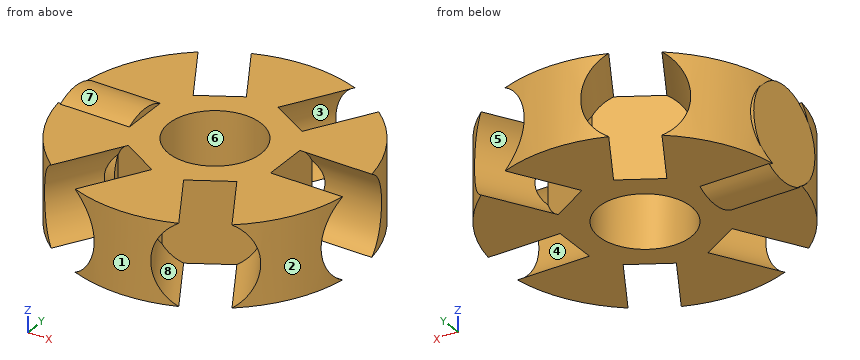
```python
from build123d import *

# Parameters (mm, degrees)
SKETCH1_R           = 12.5
SKETCH1_R_2         = 4
BOSS_EXTRUDE1_DEPTH = 3.5
SKETCH2_R           = 4
CUT_EXTRUDE3_DEPTH  = 6.4
CIRPATTERN1_COUNT   = 6
SKETCH3_R           = 4.05
BOSS_EXTRUDE2_DEPTH = 6


with BuildPart() as part:
    # Sketch1 → Boss-Extrude1 (new body, symmetric)
    with BuildSketch(Plane.XY):
        Circle(SKETCH1_R)
        Circle(SKETCH1_R_2, mode=Mode.SUBTRACT)
    extrude(amount=BOSS_EXTRUDE1_DEPTH, both=True)

    # Sketch2 → Cut-Extrude3 (cut)
    with BuildSketch(Plane(origin=(-12.5, -17.193061184, 0), x_dir=(0, -1, 0), z_dir=(1, 0, 0))):
        with Locations((-17.193061184, 0)):
            Circle(SKETCH2_R)
    cut_extrude3 = extrude(amount=CUT_EXTRUDE3_DEPTH, mode=Mode.SUBTRACT)

    # CirPattern1: Cut-Extrude3 ×6 about axis
    cirpattern1_axis = Axis((0, 0, 0), (0, 0, 1))
    for i in range(1, CIRPATTERN1_COUNT):
        add(cut_extrude3.rotate(cirpattern1_axis, i * 360 / CIRPATTERN1_COUNT), mode=Mode.SUBTRACT)

    # Sketch3 → Boss-Extrude2 (add)
    with BuildSketch(Plane(origin=(-6.1, 0, 0), x_dir=(0, -1, 0), z_dir=(-1, 0, 0))):
        Circle(SKETCH3_R)
    extrude(amount=BOSS_EXTRUDE2_DEPTH)


solid = part.part
```
The model under review builds one solid part; all positions refer to its coordinate system, in mm. Face numbers are marked on the shaded views. A direction names the side the tool comes from. Round coordinates to 2 decimals unless told otherwise and drop trailing zeros. Loops run counter-clockwise (first coordinate to the right, second up) from the corner with the lowest first, then second, coordinate; pieces in that order, holes last.
1) Consider section A-A on y = 0. State the section outline as (x, z) points.
Values follow:
outline: (-12.1, -4.05) - (-6.1, -4.05) - (-6.1, -3.5) - (-4, -3.5) - (-4, 3.5) - (-6.1, 3.5) - (-6.1, 4.05) - (-12.1, 4.05) - close; (4, -3.5) - (6.1, -3.5) - (6.1, 3.5) - (4, 3.5) - close
2) The part is to be moulded in two halves that separate along Z. For the marked faces 6, 7 and 8, say which applies: pulls with the +Z half, pulls with the -Z half, needs draft (parallel to the pull), parting line crosses it, or undercut.
Values follow:
face 6: needs draft
face 7: pulls with the +Z half
face 8: undercut
3) Wall thickness on line 1 along X through (y, z) = (-6.25, 3.25); line 2 along Z through (x, y) = (0.5, 7); line 3 along Z through (x, y) = (-9.5, -2.25): over which ranges is each line inside the solid? List them lowest first.
Values follow:
line 1: x = -10.83 to -6.3, -1.37 to 1.37, 6.3 to 10.83
line 2: z = -3.5 to -2.57, 2.57 to 3.5
line 3: z = -3.5 to 3.5
4) Consider section C-C on z = 3. State the section outline as (x, y) points.
Values follow:
outline: (-12.22, -2.65) arc R12.5 ccw to (-8.4, -9.26) - (-5.34, -3.96) - (-0.76, -6.61) - (-3.82, -11.9) arc R12.5 ccw to (3.82, -11.9) - (0.76, -6.61) - (5.34, -3.96) - (8.4, -9.26) arc R12.5 ccw to (12.22, -2.65) - (6.1, -2.65) - (6.1, 2.65) - (12.22, 2.65) arc R12.5 ccw to (8.4, 9.26) - (5.34, 3.96) - (0.76, 6.61) - (3.82, 11.9) arc R12.5 ccw to (-3.82, 11.9) - (-0.76, 6.61) - (-5.34, 3.96) - (-8.4, 9.26) arc R12.5 ccw to (-12.22, 2.65) - (-12.1, 2.65) - (-12.1, -2.65) - close; hole circle Ø8 at (0, 0)
5) Clearance check with flat-ended pins moving along their axes: P1, Ø3.5, axis at y = 1.5, z = 1, coming from the +X side; P2, Ø4, axis at x = -4, y = -7, coming from the +Z side; P3, Ø3, axis at y = 6.5, z = 2.5, coming from the +X side. State where each tip first meets the part, or that it passes through.
Values follow:
P1: stops at x = 6.1
P2: stops at z = 3.5
P3: stops at x = 11.46
6) Tool access review of the marked faces 1, 2, 3, 4 and 5: name each direction out of +Z, -Z, +X, -X, +Y, -Y from which nothing blocks a thin tool from reaching the whole face with its end or side.
Values follow:
face 1: +Z, -Z, -Y
face 2: +Z, -Z, +X, -Y
face 3: none
face 4: +X
face 5: +Y
7) Consider section B-B on z = 0.5. Give the number of separate pieces and of enclosed holes in the cut face, then the cut area to 3 significant figures.
Values follow:
separate pieces: 5
enclosed holes: 1
area: 196 mm2
